Print and shaded views of the part. All mm, measured from the part's lowest x, y and z. A direction names the side the tool comes from. Coordinates: 2 decimals unless noted, no trailing zeros. Loops run counter-clockwise (first coordinate to the right, second up) from the corner with the lowest first, then second, coordinate; pieces in that order, holes last. Notation, with made-up numbers: M 3,-14.75 L 24,-14.75 A16 cw 24,16.25 Z; hole C 45.5,1 d6. An arc over 180 degrees is marked long. Use a Markdown table: item, result. Add a question column.
1) Tool access for the marked faces 1 and 2: list every direction of +Z, -Z, +X, -X, +Y, -Y with a clear straight run to the whole face (end or side of a thin tool).
2) Band-saw the part on D-D (y = 2.25). List the corners of the cut face in (x, z).
3) Pull direction Z, two halves, no side cores. Call the marked faces 3, 4, 5 and 6: released by +Z, released by -Z, zero draft, split by the parting line, or undercut.
4) Wall check: probe 1 along X at (y, z) = (27.4, 6.35); probe 2 along Y at (x, z) = (11, 4) (1 decimal); probe 3 along Z at (x, y) = (13.97, 26.55). Give the ranges that are in metal, low to high. Write a range as from..to.
5) Band-saw the part on A-A (z = 6.35). List the corners of the cut face in (x, y) (1 decimal).
6) Pin check, flat tips, straight feed: pin 1 Ø10 at (x, z) = (24, 4.5) entering from -Y; pin 2 Ø3 at (x, y) = (8.5, 14) entering from +Z. Stop position of each tip, or through.
7) Band-saw the part on B-B (x = 26.67). List the corners of the cut face in (y, z) (1 decimal).
8) Band-saw the part on C-C (x = 20). List the corners of the cut face in (y, z) (1 decimal).
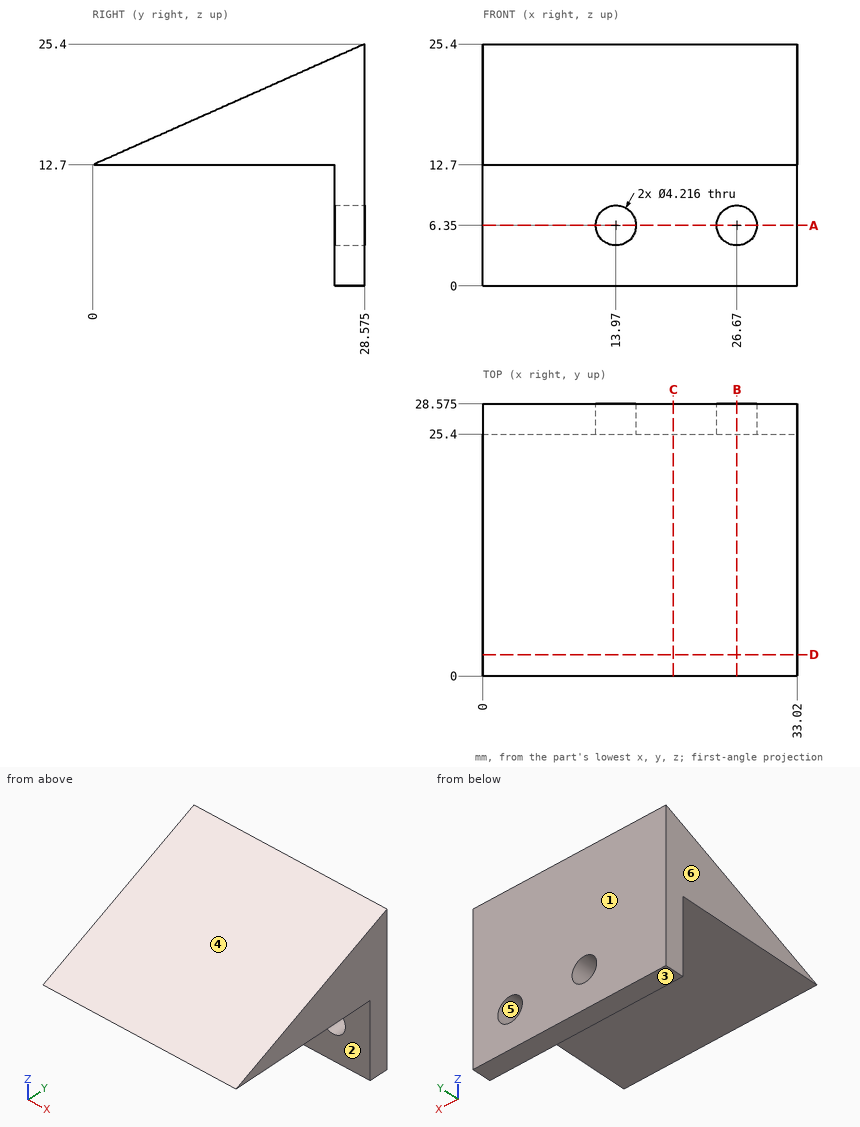
Entries:
| question | item | result |
|---|---|---|
| 1 | face 1 | +Z, -Z, +X, -X, +Y |
| 1 | face 2 | -Z, +X, -X, -Y |
| 2 | outline | M 0,12.7 L 33.02,12.7 L 33.02,13.7 L 0,13.7 Z |
| 3 | face 3 | released by -Z |
| 3 | face 4 | released by +Z |
| 3 | face 5 | undercut |
| 3 | face 6 | zero draft |
| 4 | probe 1 | 0..11.86, 16.08..24.56, 28.78..33.02 |
| 4 | probe 2 | 25.4..28.6 |
| 4 | probe 3 | 0..4.24, 8.46..24.5 |
| 5 | outline | M 0,25.4 L 11.9,25.4 L 11.9,28.6 L 0,28.6 Z; M 16.1,25.4 L 24.6,25.4 L 24.6,28.6 L 16.1,28.6 Z; M 28.8,25.4 L 33,25.4 L 33,28.6 L 28.8,28.6 Z |
| 6 | pin 1 | y = 25.4 |
| 6 | pin 2 | z = 19.59 |
| 7 | outline | M 0,12.7 L 25.4,12.7 L 25.4,8.5 L 28.6,8.5 L 28.6,25.4 Z; M 25.4,0 L 28.6,0 L 28.6,4.2 L 25.4,4.2 Z |
| 8 | outline | M 0,12.7 L 25.4,12.7 L 25.4,0 L 28.6,0 L 28.6,25.4 Z |
